Part model, mm, in its own coordinate system. A direction names the side the tool comes from. Give positions to 0.01 mm unless a question says otherwise; leave off trailing zeros. Order: outer loops, then holes, each group sorted by start corner. A loop starts at its lowest first (then second) coordinate and runs counter-clockwise, first axis right, second up. Notation, with made-up numbers: M -10.5,-27.5 L 30.5,-27.5 A20 cw 30.5,3.5 Z; hole C 77.25,59 d4. An arc over 180 degrees is marked long. Answer as a JSON object with one key per item and string values.
from build123d import *

# Parameters (mm, degrees)
SKETCH_3_W               = 45
SKETCH_3_H               = 45
EXTRUDE_1_DEPTH          = 10
EXTRUDE_START            = -38.5
SKETCH_4_W               = 19.8
SKETCH_4_H               = 22
EXTRUDE_2_DEPTH          = 32
SKETCH_5_W               = 16.3
SKETCH_5_H               = 19.8
CUT_EXTRUDE_1_DEPTH      = 22
SKETCH_6_R               = 6
EXTRUDE_3_DEPTH          = 19.5
CUT_EXTRUDE_START        = -3.1
SKETCH_7_R               = 6
SKETCH_7_R_2             = 5.4
CUT_EXTRUDE_3_DEPTH      = 0.93
SKETCH_8_R               = 3
CUT_EXTRUDE_4_DEPTH      = 39.684622268
MIRROR_4_COPY_1_SKETCH_R = 3
MIRROR_4_COPY_1_DEPTH    = 39.684622268
EXTRUDE_4_DEPTH          = 0.93
FILLET_1_R               = 2.25
FILLET_2_R               = 1.98
CHAMFER_1_SIZE           = 0.62


with BuildPart() as part:
    # 草图3 → 凸台-拉伸1 (new body)
    with BuildSketch(Plane(origin=(0, 0, 0), x_dir=(1, 0, 0), z_dir=(0, 1, 0))):
        Rectangle(SKETCH_3_W, SKETCH_3_H)
    extrude(amount=EXTRUDE_1_DEPTH)

    # 草图4 → 凸台-拉伸2 (add)
    with BuildSketch(Plane(origin=(22.5, 0, 0), x_dir=(0, 0, -1), z_dir=(1, 0, 0)).offset(EXTRUDE_START)):
        with Locations((0, 21)):
            Rectangle(SKETCH_4_W, SKETCH_4_H)
    extrude(amount=EXTRUDE_2_DEPTH)

    # 草图5 → 切除-拉伸1 (cut)
    with BuildSketch(Plane(origin=(0, 10, 0), x_dir=(-1, 0, 0), z_dir=(0, 1, 0))):
        Rectangle(SKETCH_5_W, SKETCH_5_H)
    extrude(amount=CUT_EXTRUDE_1_DEPTH, mode=Mode.SUBTRACT)

    # 草图6 → 凸台-拉伸3 (add)
    with BuildSketch(Plane(origin=(0, 0, 0), x_dir=(0, 0, -1), z_dir=(1, 0, 0))):
        with Locations(Location((0, 19, 0), (0, 0, 180))):
            Circle(SKETCH_6_R)
    extrude_3 = extrude(amount=EXTRUDE_3_DEPTH)

    # 镜向1: 凸台-拉伸3 across plane
    add(extrude_3.mirror(Plane(origin=(0, 0, 0), x_dir=(0, 0, 1), z_dir=(1, 0, 0))))

    # 草图7 → 切除-拉伸3 (cut)
    with BuildSketch(Plane(origin=(19.5, 0, 0), x_dir=(0, 0, -1), z_dir=(1, 0, 0)).offset(CUT_EXTRUDE_START)):
        with Locations(Location((0, 19, 0), (0, 0, 180))):
            Circle(SKETCH_7_R)
        with Locations((0, 19)):
            Circle(SKETCH_7_R_2, mode=Mode.SUBTRACT)
    cut_extrude_3 = extrude(amount=CUT_EXTRUDE_3_DEPTH, mode=Mode.SUBTRACT)

    # 镜向2: 切除-拉伸3 across plane
    add(cut_extrude_3.mirror(Plane(origin=(0, 0, 0), x_dir=(0, 0, 1), z_dir=(1, 0, 0))), mode=Mode.SUBTRACT)

    # 草图8 → 切除-拉伸4 (cut, through all)
    with BuildSketch(Plane(origin=(0, 10, 0), x_dir=(1, 0, 0), z_dir=(0, 1, 0))):
        with Locations(Location((-16.5, 16.5, 0), (0, 0, 270))):
            Circle(SKETCH_8_R)
    cut_extrude_4 = extrude(amount=-CUT_EXTRUDE_4_DEPTH, mode=Mode.SUBTRACT)

    # 镜向3: 切除-拉伸4 across plane
    add(cut_extrude_4.mirror(Plane(origin=(0, 0, 0), x_dir=(0, 0, 1), z_dir=(1, 0, 0))), mode=Mode.SUBTRACT)

    # 镜向4: 切除-拉伸4 across plane
    add(cut_extrude_4.mirror(Plane.XY), mode=Mode.SUBTRACT)

    # 镜向4 copy 1 sketch → 镜向4 copy 1 (cut, through all)
    with BuildSketch(Plane(origin=(0, 10, 0), x_dir=(-1, 0, 0), z_dir=(0, 1, 0))):
        with Locations(Location((-16.5, 16.5, 0), (0, 0, 270))):
            Circle(MIRROR_4_COPY_1_SKETCH_R)
    extrude(amount=-MIRROR_4_COPY_1_DEPTH, mode=Mode.SUBTRACT)

    # 草图9 → 凸台-拉伸4 (add)
    with BuildSketch(Plane(origin=(16.4, 0, 0), x_dir=(0, 0, -1), z_dir=(1, 0, 0))):
        with BuildLine():
            Line((0, 19), (-3.6, 12.764617093))
            ThreePointArc((-3.6, 12.764617093), (0, 26.2), (3.6, 12.764617093))
            Line((3.6, 12.764617093), (0, 19))
        make_face()
    extrude_4 = extrude(amount=EXTRUDE_4_DEPTH)

    # 镜向5: 凸台-拉伸4 across plane
    add(extrude_4.mirror(Plane(origin=(0, 0, 0), x_dir=(0, 0, 1), z_dir=(1, 0, 0))))

    # 圆角1
    fillet_1_edges = [part.edges().sort_by_distance(p)[0] for p in [
        (-22.5, 5, 22.5),
        (-22.5, 5, -22.5),
        (22.5, 5, -22.5),
        (22.5, 5, 22.5),
    ]]
    fillet(fillet_1_edges, radius=FILLET_1_R)

    # 圆角2
    fillet_2_edges = [part.edges().sort_by_distance(p)[0] for p in [
        (12.075, 32, -9.9),
        (12.075, 32, 9.9),
        (-12.075, 32, 9.9),
        (-12.075, 32, -9.9),
    ]]
    fillet(fillet_2_edges, radius=FILLET_2_R)

    # 倒角1
    chamfer_1_edges = [part.edges().sort_by_distance(p)[0] for p in [
        (19.5, 19, -6),
        (-19.5, 19, -6),
    ]]
    chamfer(chamfer_1_edges, length=CHAMFER_1_SIZE)


solid = part.part
1. Cut at A-A on x = 4. Give the cut face in (y, z).
Worked answers:
{"outline": "M 0,-22.5 L 10,-22.5 L 10,22.5 L 0,22.5 Z; C 19,0 d12"}
2. Cut at B-B on z = 16.5. Give the cut face in (x, y).
Worked answers:
{"outline": "M -22.5,0 L -19.5,0 L -19.5,10 L -22.5,10 Z; M -13.5,0 L 13.5,0 L 13.5,10 L -13.5,10 Z; M 19.5,0 L 22.5,0 L 22.5,10 L 19.5,10 Z"}
3. Cut at D-D on z = -15. Give the cut face in (x, y).
Worked answers:
{"outline": "M -22.5,0 L -19.1,0 L -19.1,10 L -22.5,10 Z; M -13.9,0 L 13.9,0 L 13.9,10 L -13.9,10 Z; M 19.1,0 L 22.5,0 L 22.5,10 L 19.1,10 Z"}
4. Pin check, flat tips, straight feed: P1, Ø1.5, axis at y = 14, z = 0, coming from the -X side; P2, Ø4, axis at y = 14.5, z = -5, coming from the +X side; P3, Ø8, axis at x = 0.5, z = 18, coming from the +Y side. Stop position of each tip, or through.
Worked answers:
{"P1": "stops at x = -19.5", "P2": "stops at x = 19.5", "P3": "stops at y = 10"}
5. Two-plate mould, pull along Z, no slides. Class faces 1 (the flat face through (19.5, 19, 0)), 2 (the cylindrical face through (-16.858, 26.195, 0.264)), 3 (the cylindrical face through (19.43, 5.07, 17.15)): +Z half, -Z half, draft (parallel to the pull), parting line (faces both ways), or undercut.
Worked answers:
{"face 1": "draft", "face 2": "parting line", "face 3": "undercut"}
6. Probe line 1 along X through (y, z) = (5.75, 16.5); line 2 along X through (y, z) = (12, -9.5). List the from-to ranges inside material, lowest first.
Worked answers:
{"line 1": "x = -22.5 to -19.5, -13.5 to 13.5, 19.5 to 22.5", "line 2": "x = -16 to -8.15, 8.15 to 16"}
7. Cut at C-C on x = -11. Give the cut face in (y, z).
Worked answers:
{"outline": "M 0,-22.5 L 10,-22.5 L 10,-9.9 L 30.02,-9.9 A1.98 ccw 32,-7.92 L 32,7.92 A1.98 ccw 30.02,9.9 L 10,9.9 L 10,22.5 L 0,22.5 Z"}
8. Which spindle directions (+Z, -Z, +X, -X, +Y, -Y) get a long thin tool onto all of the face, cutting with end or side? Do faces 4 (the flat face through (-19.5, 19, 0)), 5 (the flat face through (-12, 20, 9.9)), 6 (the flat face through (-16.4, 13.4, 0)), 7 (the flat face through (-17.33, 25.5, 0)). Say none if no direction does.
Worked answers:
{"face 4": "+Z, -Z, -X, +Y", "face 5": "+Z, +X, -X, +Y", "face 6": "none", "face 7": "-X"}
